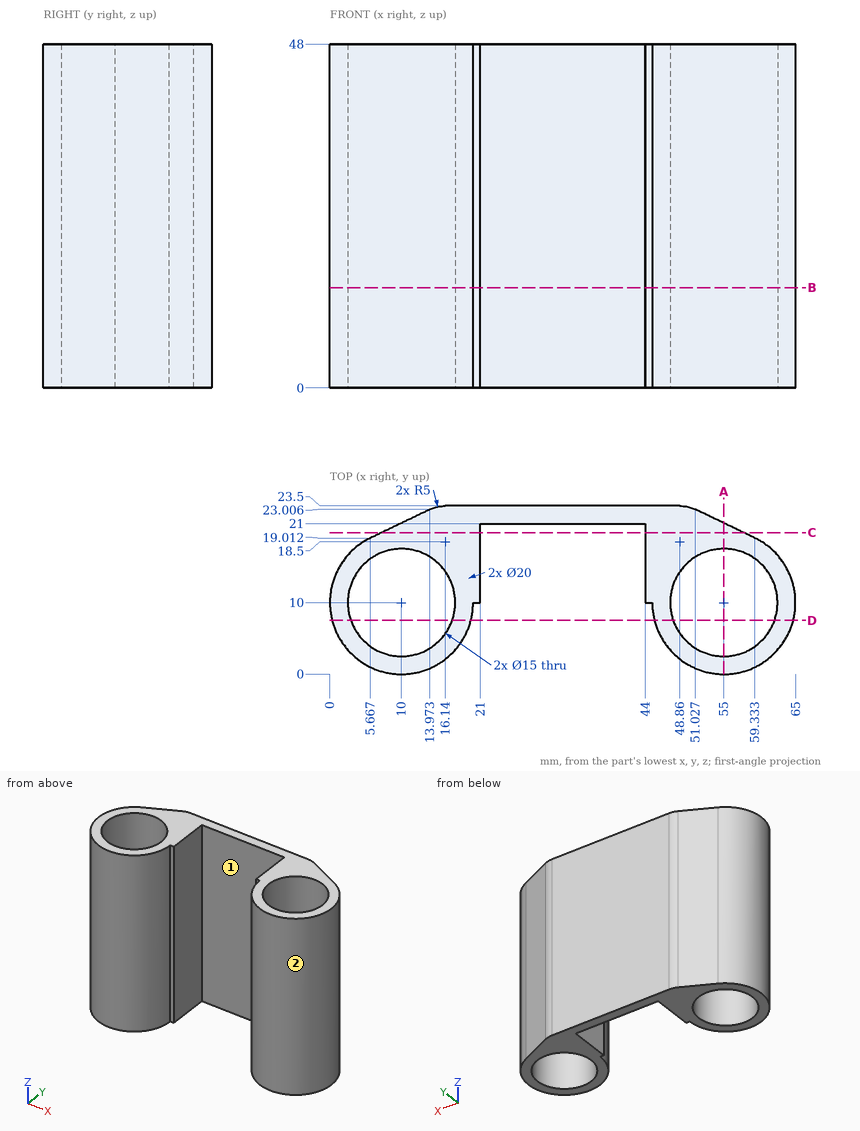
Check sheet for the drawn part. Datum: minimum x, y, z corner. Units: mm. A direction names the side the tool comes from. Round coordinates to 2 decimals unless told otherwise and drop trailing zeros. Order: outer loops, then holes, each group sorted by start corner. A loop starts at its lowest first (then second) coordinate and runs counter-clockwise, first axis right, second up. Notation, with made-up numbers: (37.25, 36.5) -> (63.25, 36.5) arc R20 cw to (63.25, 71.5) -> close; hole circle Ø10 at (5, -14.5). An arc over 180 degrees is marked (long way). Put each result on its own line as item: value. Start each with the question number.
(1) Material ranges on line 1 along X through (y, z) = (7.75, 3.5) (1 decimal); line 2 along X through (y, z) = (13.75, 6) (1 decimal); line 3 along Y through (x, z) = (27.5, 28), recorded low to high.
(2) Section check D-D (y = 7.5). Enter the section's corners in (x, z).
(3) Section check B-B (z = 14). Enter the section's corners in (x, y).
(4) Section check C-C (y = 19.75). Enter the section's corners in (x, z).
(5) Depth check by flat-ended pin: pin 1 Ø3.5 at (y, z) = (15.5, 33) entering from -X; pin 2 Ø0.5 at (x, z) = (20.5, 12.5) entering from -Y; pin 3 Ø10 at (x, z) = (27, 17) entering from -Y; pin 4 Ø9 at (x, y) = (55, 10) entering from +Z. Enter the tip coordinate at first touch or a pass-through.
(6) Section check A-A (x = 55). Enter the section's corners in (y, z).
(7) Tool access check on the marked faces 1 and 2. Record the directions out of +Z, -Z, +X, -X, +Y, -Y that give a thin tool (end or side, any length) a straight path to the whole face; none if there is none.
Completed:
1. line 1: x = 0.3 to 2.8, 17.2 to 19.7, 45.3 to 47.8, 62.2 to 64.7
1. line 2: x = 0.7 to 3.5, 16.5 to 21, 44 to 48.5, 61.5 to 64.3
1. line 3: y = 21 to 23.5
2. outline: (0.32, 0) -> (2.93, 0) -> (2.93, 48) -> (0.32, 48) -> close; (17.07, 0) -> (19.68, 0) -> (19.68, 48) -> (17.07, 48) -> close; (45.32, 0) -> (47.93, 0) -> (47.93, 48) -> (45.32, 48) -> close; (62.07, 0) -> (64.68, 0) -> (64.68, 48) -> (62.07, 48) -> close
3. outline: (5.67, 19.01) arc R10 ccw (long way) to (20, 10) -> (21, 10) -> (21, 21) -> (44, 21) -> (44, 10) -> (45, 10) arc R10 ccw (long way) to (59.33, 19.01) -> (51.03, 23.01) arc R5 ccw to (48.86, 23.5) -> (16.14, 23.5) arc R5 ccw to (13.97, 23.01) -> close; hole circle Ø15 at (10, 10); hole circle Ø15 at (55, 10)
4. outline: (7.2, 0) -> (21, 0) -> (21, 48) -> (7.2, 48) -> close; (44, 0) -> (57.8, 0) -> (57.8, 48) -> (44, 48) -> close
5. pin 1: stops at x = 0.73
5. pin 2: stops at y = 10
5. pin 3: stops at y = 21
5. pin 4: passes through
6. outline: (0, 0) -> (2.5, 0) -> (2.5, 48) -> (0, 48) -> close; (17.5, 0) -> (21.1, 0) -> (21.1, 48) -> (17.5, 48) -> close
7. face 1: +Z, -Z, -Y
7. face 2: +Z, -Z
